Geometry check sheet. Reference: the model listing, model coordinates, mm. A direction names the side the tool comes from. Coordinates: 2 decimals unless noted, no trailing zeros. Write each loop counter-clockwise with the first axis right and the second up, starting at its lowest first coordinate (ties: lowest second). Pieces come first, ordered by that corner, then holes. Notation, with made-up numbers: (32.25, 38.25) -> (41.25, 38.25) arc R23 cw to (41.25, 69.25) -> close; hole circle Ø4 at (65.5, 30). An arc over 180 degrees is marked (long way). One line per question, with ' | ' between items.
```python
from build123d import *

# Parameters (mm, degrees)
SKETCH_1_R                  = 50
EXTRUDE_1_DEPTH             = 4
HOLE_WIZARD_M41_D           = 4.5
HOLE_WIZARD_M41_CSINK_D     = 5
HOLE_WIZARD_M41_CSINK_ANGLE = 90
CUT_EXTRUDE_1_DEPTH         = 71.823724839
SKETCH_5_R                  = 53
SKETCH_5_R_2                = 50
EXTRUDE_2_DEPTH             = 25
EXTRUDE_3_REACH             = 123.12
EXTRUDE_3_END_RADIUS        = 50
SKETCH_6_R                  = 15
EXTRUDE_3_DIRECTION_2_DEPTH = 12


with BuildPart() as part:
    # Эскиз1 → Бобышка-Вытянуть1 (new body)
    with BuildSketch(Plane(origin=(0, 0, 0), x_dir=(1, 0, 0), z_dir=(0, 1, 0))):
        with Locations(Location((0, 0, 0), (0, 0, 270))):
            Circle(SKETCH_1_R)
    extrude(amount=EXTRUDE_1_DEPTH)

    # Отверстие с зазором M41 (through all)
    with Locations(Plane(origin=(0, 0, 0), x_dir=(-1, 0, 0), z_dir=(0, -1, 0))):
        with Locations((-21.25, 36.806079661), (0, 42.5), (21.25, 36.806079661), (36.806079661, 21.25), (42.5, 0), (36.806079661, -21.25), (21.25, -36.806079661), (0, -42.5), (-21.25, -36.806079661), (-36.806079661, -21.25), (-42.5, 0), (-36.806079661, 21.25)):
            CounterSinkHole(HOLE_WIZARD_M41_D / 2, HOLE_WIZARD_M41_CSINK_D / 2, counter_sink_angle=HOLE_WIZARD_M41_CSINK_ANGLE)

    # Эскиз4 → Вырез-Вытянуть1 (cut, through all)
    with BuildSketch(Plane.XZ):
        with BuildLine():
            Line((11.970705016, 32.889241728), (8.550503583, 23.49231552))
            ThreePointArc((8.550503583, 23.49231552), (12.5, 21.650635095), (16.069690242, 19.151111078))
            Line((16.069690242, 19.151111078), (22.497566339, 26.811555509))
            ThreePointArc((22.497566339, 26.811555509), (17.5, 30.310889132), (11.970705016, 32.889241728))
        make_face()
        with BuildLine():
            Line((-6.077686218, 34.468271355), (-4.341204442, 24.620193825))
            ThreePointArc((-4.341204442, 24.620193825), (0, 25), (4.341204442, 24.620193825))
            Line((4.341204442, 24.620193825), (6.077686218, 34.468271355))
            ThreePointArc((6.077686218, 34.468271355), (0, 35), (-6.077686218, 34.468271355))
        make_face()
        with BuildLine():
            Line((32.889241728, -11.970705016), (23.49231552, -8.550503583))
            ThreePointArc((23.49231552, -8.550503583), (21.650635095, -12.5), (19.151111078, -16.069690242))
            Line((19.151111078, -16.069690242), (26.811555509, -22.497566339))
            ThreePointArc((26.811555509, -22.497566339), (30.310889132, -17.5), (32.889241728, -11.970705016))
        make_face()
        with BuildLine():
            Line((34.468271355, 6.077686218), (24.620193825, 4.341204442))
            ThreePointArc((24.620193825, 4.341204442), (25, 0), (24.620193825, -4.341204442))
            Line((24.620193825, -4.341204442), (34.468271355, -6.077686218))
            ThreePointArc((34.468271355, -6.077686218), (35, 0), (34.468271355, 6.077686218))
        make_face()
        with BuildLine():
            Line((26.811555509, 22.497566339), (19.151111078, 16.069690242))
            ThreePointArc((19.151111078, 16.069690242), (21.650635095, 12.5), (23.49231552, 8.550503583))
            Line((23.49231552, 8.550503583), (32.889241728, 11.970705016))
            ThreePointArc((32.889241728, 11.970705016), (30.310889132, 17.5), (26.811555509, 22.497566339))
        make_face()
        with BuildLine():
            Line((-11.970705016, -32.889241728), (-8.550503583, -23.49231552))
            ThreePointArc((-8.550503583, -23.49231552), (-12.5, -21.650635095), (-16.069690242, -19.151111078))
            Line((-16.069690242, -19.151111078), (-22.497566339, -26.811555509))
            ThreePointArc((-22.497566339, -26.811555509), (-17.5, -30.310889132), (-11.970705016, -32.889241728))
        make_face()
        with BuildLine():
            Line((6.077686218, -34.468271355), (4.341204442, -24.620193825))
            ThreePointArc((4.341204442, -24.620193825), (0, -25), (-4.341204442, -24.620193825))
            Line((-4.341204442, -24.620193825), (-6.077686218, -34.468271355))
            ThreePointArc((-6.077686218, -34.468271355), (0, -35), (6.077686218, -34.468271355))
        make_face()
        with BuildLine():
            Line((22.497566339, -26.811555509), (16.069690242, -19.151111078))
            ThreePointArc((16.069690242, -19.151111078), (12.5, -21.650635095), (8.550503583, -23.49231552))
            Line((8.550503583, -23.49231552), (11.970705016, -32.889241728))
            ThreePointArc((11.970705016, -32.889241728), (17.5, -30.310889132), (22.497566339, -26.811555509))
        make_face()
        with BuildLine():
            Line((-22.497566339, 26.811555509), (-16.069690242, 19.151111078))
            ThreePointArc((-16.069690242, 19.151111078), (-12.5, 21.650635095), (-8.550503583, 23.49231552))
            Line((-8.550503583, 23.49231552), (-11.970705016, 32.889241728))
            ThreePointArc((-11.970705016, 32.889241728), (-17.5, 30.310889132), (-22.497566339, 26.811555509))
        make_face()
        with BuildLine():
            Line((-32.889241728, 11.970705016), (-23.49231552, 8.550503583))
            ThreePointArc((-23.49231552, 8.550503583), (-21.650635095, 12.5), (-19.151111078, 16.069690242))
            Line((-19.151111078, 16.069690242), (-26.811555509, 22.497566339))
            ThreePointArc((-26.811555509, 22.497566339), (-30.310889132, 17.5), (-32.889241728, 11.970705016))
        make_face()
        with BuildLine():
            Line((-34.468271355, -6.077686218), (-24.620193825, -4.341204442))
            ThreePointArc((-24.620193825, -4.341204442), (-25, 0), (-24.620193825, 4.341204442))
            Line((-24.620193825, 4.341204442), (-34.468271355, 6.077686218))
            ThreePointArc((-34.468271355, 6.077686218), (-35, 0), (-34.468271355, -6.077686218))
        make_face()
        with BuildLine():
            Line((-26.811555509, -22.497566339), (-19.151111078, -16.069690242))
            ThreePointArc((-19.151111078, -16.069690242), (-21.650635095, -12.5), (-23.49231552, -8.550503583))
            Line((-23.49231552, -8.550503583), (-32.889241728, -11.970705016))
            ThreePointArc((-32.889241728, -11.970705016), (-30.310889132, -17.5), (-26.811555509, -22.497566339))
        make_face()
    extrude(amount=-CUT_EXTRUDE_1_DEPTH, mode=Mode.SUBTRACT)

    # Эскиз5 → Бобышка-Вытянуть2 (add)
    with BuildSketch(Plane.XZ):
        with Locations(Location((0, 0, 0), (0, 0, 270))):
            Circle(SKETCH_5_R)
        with Locations(Location((0, 0, 0), (0, 0, 270))):
            Circle(SKETCH_5_R_2, mode=Mode.SUBTRACT)
    extrude(amount=-EXTRUDE_2_DEPTH)

    # Бобышка-Вытянуть3: up to this cylinder (the profile starts outside it)
    extrude_3_end = Plane(origin=(0, 20, 0), z_dir=(0, -1, 0)) * Cylinder(EXTRUDE_3_END_RADIUS, 347.24, mode=Mode.PRIVATE)
    # Эскиз6 → Бобышка-Вытянуть3 (add, up to the surface)
    with BuildSketch(Plane(origin=(0, 0, -53), x_dir=(-1, 0, 0), z_dir=(0, 0, -1)), mode=Mode.PRIVATE) as extrude_3_sk1:
        with Locations(Location((0, 20, 0), (0, 0, 270))):
            Circle(SKETCH_6_R)
    extrude_3_tool1 = extrude(extrude_3_sk1.sketch, amount=-EXTRUDE_3_REACH, mode=Mode.PRIVATE) - extrude_3_end
    add(extrude_3_tool1.solids().sort_by_distance((0, 20, -53))[0])

    # Эскиз6 → Бобышка-Вытянуть3 direction 2 (add)
    with BuildSketch(Plane(origin=(0, 0, -53), x_dir=(-1, 0, 0), z_dir=(0, 0, -1))):
        with Locations(Location((0, 20, 0), (0, 0, 270))):
            Circle(SKETCH_6_R)
    extrude(amount=EXTRUDE_3_DIRECTION_2_DEPTH)

    # Фаска1
    # the kernel refuses this chamfer: 4.922263446, 3 mm, written as the material it adds along each edge
    with BuildSketch(Plane(origin=(-14.142135624, 25, -35.782012711), x_dir=(0.4567037987045211, 0.8896188173868965, 0), z_dir=(0, 0, -1))) as chamfer_1_piece_1_section:
        with BuildLine():
            Line((2.315673344, 0), (-2.283325225, -4.302139097))
            Line((-2.283325225, -4.302139097), (-2.370903989, -4.257178768))
            ThreePointArc((-2.370903989, -4.257178768), (-1.199667859, -2.121291383), (-0.087578764, 0.044960328))
            Line((-0.087578764, 0.044960328), (0.013196083, 0.097556826))
            ThreePointArc((0.013196083, 0.097556826), (1.157121783, -0.012460261), (2.31461529, 0.098439583))
            Line((2.31461529, 0.098439583), (2.315673344, 0))
        make_face()
    chamfer_1_piece_1 = extrude(amount=27.472660966, mode=Mode.PRIVATE)
    chamfer_1_piece_1 = chamfer_1_piece_1 & Plane(origin=(0, 25.614085428, 0), x_dir=(0, 0, -1), z_dir=(0, -1, 0)) * Cylinder(53, 73, mode=Mode.PRIVATE)
    chamfer_1_piece_1 = chamfer_1_piece_1 - Plane(origin=(0, 25.614085428, 0), x_dir=(0, 0, -1), z_dir=(0, -1, 0)) * Cylinder(50, 73, mode=Mode.PRIVATE)
    add(chamfer_1_piece_1)
    with BuildSketch(Plane(origin=(14.142135624, 25, -35.782012711), x_dir=(-0.45670379870452116, 0.8896188173868965, 0), z_dir=(0, 0, -1))) as chamfer_1_piece_2_section:
        with BuildLine():
            Line((2.315673344, 0), (-2.283325225, 4.302139097))
            Line((-2.283325225, 4.302139097), (-2.370903989, 4.257178768))
            ThreePointArc((-2.370903989, 4.257178768), (-1.199667859, 2.121291383), (-0.087578764, -0.044960328))
            Line((-0.087578764, -0.044960328), (0.013196083, -0.097556826))
            ThreePointArc((0.013196083, -0.097556826), (1.157121783, 0.012460261), (2.31461529, -0.098439583))
            Line((2.31461529, -0.098439583), (2.315673344, 0))
        make_face()
    chamfer_1_piece_2 = extrude(amount=27.472660966, mode=Mode.PRIVATE)
    chamfer_1_piece_2 = chamfer_1_piece_2 & Plane(origin=(0, 25.614085428, 0), x_dir=(0, 0, -1), z_dir=(0, -1, 0)) * Cylinder(53, 73, mode=Mode.PRIVATE)
    chamfer_1_piece_2 = chamfer_1_piece_2 - Plane(origin=(0, 25.614085428, 0), x_dir=(0, 0, -1), z_dir=(0, -1, 0)) * Cylinder(50, 73, mode=Mode.PRIVATE)
    add(chamfer_1_piece_2)


solid = part.part
```
(1) Cross-section at A-A (x = 0). Count the separate pieces of the cut face and the enclosed holes in it, plus the area to 3 significant figures.
Answers below:
separate pieces: 5 | enclosed holes: 0 | area: 824 mm²
(2) Cross-section at D-D (z = 42.5). Record the cut outline in (x, y).
Answers below:
outline: (-31.67, 0) -> (-2.5, 0) -> (-2.25, 0.25) -> (-2.25, 4) -> (-26.34, 4) -> (-26.34, 25) -> (-31.67, 25) -> close; (2.25, 0.25) -> (2.5, 0) -> (31.67, 0) -> (31.67, 25) -> (26.34, 25) -> (26.34, 4) -> (2.25, 4) -> close
(3) Tool access check on faces 1 (the face through (1, 0, 1)), 2 (the face through (0, 2, 25)). Record the directions out of +Z, -Z, +X, -X, +Y, -Y that give a thin tool (end or side, any length) a straight path to the whole face; none if there is none.
Answers below:
face 1: +Z, -Z, +X, -X, -Y | face 2: +Y, -Y
(4) Cross-section at C-C (z = 14). Record the cut outline in (x, y).
Answers below:
outline: (-51.12, 0) -> (-32.08, 0) -> (-32.08, 4) -> (-48, 4) -> (-48, 25) -> (-51.12, 25) -> close; (-20.71, 0) -> (20.71, 0) -> (20.71, 4) -> (-20.71, 4) -> close; (32.08, 0) -> (51.12, 0) -> (51.12, 25) -> (48, 25) -> (48, 4) -> (32.08, 4) -> close
(5) Cross-section at B-B (z = 0). Record the cut outline in (x, y), plus the area to 3 significant figures.
Answers below:
outline: (-53, 0) -> (-45, 0) -> (-44.75, 0.25) -> (-44.75, 4) -> (-50, 4) -> (-50, 25) -> (-53, 25) -> close; (-40.25, 0.25) -> (-40, 0) -> (-35, 0) -> (-35, 4) -> (-40.25, 4) -> close; (-25, 0) -> (25, 0) -> (25, 4) -> (-25, 4) -> close; (35, 0) -> (40, 0) -> (40.25, 0.25) -> (40.25, 4) -> (35, 4) -> close; (44.75, 0.25) -> (45, 0) -> (53, 0) -> (53, 25) -> (50, 25) -> (50, 4) -> (44.75, 4) -> close | area: 434 mm²
(6) Draft check along Z on faces 3 (the face through (15.92, 13.308, -50.553)), 4 (the face through (0, 20, -65)), 5 (the face through (29.5, 2, -5.2)). Enter one of: pulls with the +Z half, pulls with the -Z half, needs draft (parallel to the pull), parting line crosses it, or undercut.
Answers below:
face 3: parting line crosses it | face 4: pulls with the -Z half | face 5: undercut
(7) Material ranges on line 1 (X direction, y = 6, z = 1); line 2 (X direction, y = 7, z = 32); line 3 (Y direction, x = 47, z = -21), recorded low to high.
Answers below:
line 1: x = -52.99 to -49.99, 49.99 to 52.99 | line 2: x = -42.25 to -38.42, 38.42 to 42.25 | line 3: y = 0 to 25
(8) Depth check by flat-ended pin: P1, Ø4, axis at y = 13.5, z = -44.5, coming from the +X side; P2, Ø5, axis at x = 36.81, z = -21.25, coming from the +Y side; P3, Ø8, axis at x = -40, y = 5, coming from the +Z side; P4, Ø6, axis at x = -21.25, z = -36.81, coming from the -Y side. Enter the tip coordinate at first touch or a pass-through.
Answers below:
P1: stops at x = 31.67 | P2: stops at y = 4 | P3: stops at z = 38.9 | P4: stops at y = 0
